Build history of the part. All positions in model axes, mm. Face numbers are marked on the shaded views. Coordinates: 2 decimals unless noted, no trailing zeros. Write each loop counter-clockwise with the first axis right and the second up, starting at its lowest first coordinate (ties: lowest second). Pieces come first, ordered by that corner, then holes. Notation, with made-up numbers: M 68,53 L 113,53 A31 cw 113,82 Z; hole C 79.5,41.5 d5. An arc over 180 degrees is marked long. Use CSV: the item, a comma, the result in double quotes. Start each with the question number.
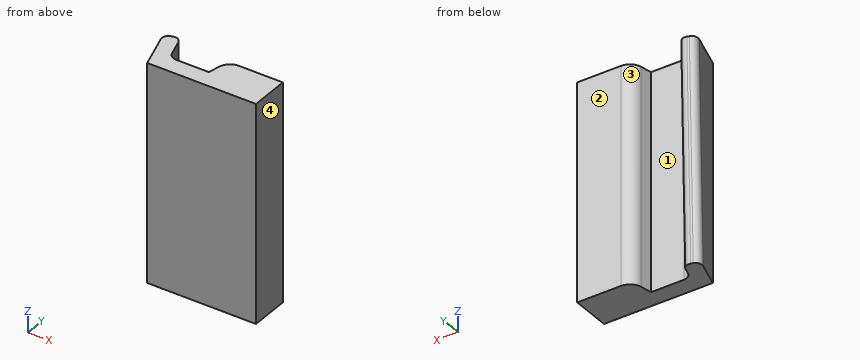
```python
from build123d import *

# Parameters (mm, degrees)
F1_DEPTH    = 50
F2_SIZE2    = 2.49999
F2_SIZE     = 49.99999
F3_T1_DEPTH = 57.5624504994
F4_R        = 2
F5_R        = 3


# Not quite as in the source:
# - a fillet or chamfer that OpenCascade refuses, or shapes differently, is made with other operations: its cross-section is extruded or revolved along the edge and cut away or added
# - a fillet or chamfer is up to 0.001 mm smaller than in the source, because OpenCascade refuses the exact size


with BuildPart() as f1:
    # F0 (on Top) → F1 (new body)
    with BuildSketch(Plane.XY):
        Polygon((-4.0792049388, 6.6941332917), (-7.4262715846, 5.6708323252), (-4.4696014276, -4), (20.5303985724, -4), (20.5303985724, 5), (8.0088521886, 5), (6.9673969943, 0), (-2.0326030057, 0), align=None)
    extrude(amount=F1_DEPTH)

    # F2 (size 50 and 2.5 in the source; OpenCascade refuses exactly that, so slightly less here)
    f2_edges = [f1.edges().sort_by_distance(p)[0] for p in [
        (-5.752738, 6.182483, 0),
    ]]
    f2_side = f1.faces().sort_by_distance((-5.752738, 6.182483, 25))[0]
    chamfer(f2_edges, length=F2_SIZE, length2=F2_SIZE2, reference=f2_side)

    # F3: fillet of radius 1.5 on 2 edges, made by hand

    # F3_s2 → F3_t1 (cut)
    with BuildSketch(Plane(origin=(-0.7893916774, 2.5819838349, 53.9993894282), x_dir=(0.956304756, 0.2923717047, 0), z_dir=(0.0146002909, -0.0477553996, -0.9987523483))):
        with BuildLine():
            ThreePointArc((-1.9437879213, -3.5879297119), (-2.3831277496, -4.6485898837), (-3.4437879213, -5.0879297119))
            Line((-3.4437879213, -5.0879297119), (-1.9437879213, -5.0879297119))
            Line((-1.9437879213, -5.0879297119), (-1.9437879213, -3.5879297119))
        make_face()
        with BuildLine():
            ThreePointArc((-3.9437879213, -5.0879297119), (-5.0044480931, -4.6485898837), (-5.4437879213, -3.5879297119))
            Line((-5.4437879213, -3.5879297119), (-5.4437879213, -5.0879297119))
            Line((-5.4437879213, -5.0879297119), (-3.9437879213, -5.0879297119))
        make_face()
    extrude(amount=F3_T1_DEPTH, mode=Mode.SUBTRACT)

    # F4
    f4_edges = [f1.edges().sort_by_distance(p)[0] for p in [
        (-2.032603, 0, 25),
    ]]
    fillet(f4_edges, radius=F4_R)

    # F5
    f5_edges = [f1.edges().sort_by_distance(p)[0] for p in [
        (8.008852, 5, 25),
    ]]
    fillet(f5_edges, radius=F5_R)


solid = f1.part
```
1. Pull direction X, two halves, no side cores. Call the marked faces 1, 2, 3 and 4: pulls with the +X half, pulls with the -X half, needs draft (parallel to the pull), parting line crosses it, or undercut.
2. Slice it at A-A (y = 0.5). List the corners of the cut face in (x, z).
3. Slice it at C-C (y = -1.75). List the corners of the cut face in (x, z).
4. Flat gauge pins, fed straight in: pin 1 (1.5 mm diameter, centred on y = 0, z = 25.5, fed in from -X); pin 2 (11 mm diameter, centred on x = 14.5, z = 18, fed in from +Y); pin 3 (10 mm diameter, centred on x = -2, z = 15, fed in from +Y); pin 4 (4 mm diameter, centred on x = 4, y = 0, fed in from -Z). Where does each tip first touch, or does it go through?
5. Drill centre lines: line 1 along Y through (x, z) = (3, 34.5); line 2 along X through (y, z) = (2.5, 32.5); line 3 along X through (y, z) = (1, 26.5). Where is each one in solid material? Low to high. Write a range as from..to.
6. Slice it at B-B (x = 18.75). List the corners of the cut face in (y, z).
Established:
1,face 1,"undercut"
1,face 2,"needs draft"
1,face 3,"undercut"
1,face 4,"pulls with the +X half"
2,outline,"M -5.85,0 L -1.88,0 L -1.88,50 L -5.85,50 Z; M 7.07,0 L 20.53,0 L 20.53,50 L 7.07,50 Z"
3,outline,"M -5.16,0 L 20.53,0 L 20.53,50 L -5.16,50 Z"
4,pin 1,"stops at x = -5.92"
4,pin 2,"stops at y = 5"
4,pin 3,"stops at y = 4.85"
4,pin 4,"stops at z = 0"
5,line 1,"y = -4..0"
5,line 2,"x = -6.46..-2.8, 7.49..20.53"
5,line 3,"x = -6..-2.28, 7.18..20.53"
6,outline,"M -4,0 L 5,0 L 5,50 L -4,50 Z"
